```python
from build123d import *

# Parameters (mm, degrees)
SALIENTE_EXTRUIR1_DEPTH = 5
CROQUIS2_W              = 5
CROQUIS2_H              = 6.5
SALIENTE_EXTRUIR3_DEPTH = 5
REDONDEO1_R             = 3
REDONDEO2_R             = 2
REDONDEO3_R             = 1
CROQUIS4_R              = 1.75
CORTAR_EXTRUIR1_DEPTH   = 2.5
CROQUIS5_R              = 1
CORTAR_EXTRUIR2_DEPTH   = 2.5
CROQUIS6_R              = 0.75
CORTAR_EXTRUIR3_DEPTH   = 5


with BuildPart() as part:
    # Croquis1 → Saliente-Extruir1 (new body)
    with BuildSketch(Plane(origin=(0, 0, 0), x_dir=(0, 0, -1), z_dir=(1, 0, 0))):
        with BuildLine():
            Line((-13, 1.5), (13, 1.5))
            ThreePointArc((13, 1.5), (14.5, 0), (13, -1.5))
            Line((13, -1.5), (-13, -1.5))
            ThreePointArc((-13, -1.5), (-14.5, 0), (-13, 1.5))
        make_face()
    extrude(amount=SALIENTE_EXTRUIR1_DEPTH)

    # Croquis2 → Saliente-Extruir3 (add)
    with BuildSketch(Plane(origin=(5, 0, 0), x_dir=(0, 0, -1), z_dir=(1, 0, 0))):
        with Locations((-13, 0)):
            Rectangle(CROQUIS2_W, CROQUIS2_H)
        with Locations((13, 0)):
            Rectangle(CROQUIS2_W, CROQUIS2_H)
    extrude(amount=SALIENTE_EXTRUIR3_DEPTH)

    # Redondeo1
    redondeo1_edges = [part.edges().sort_by_distance(p)[0] for p in [
        (10, 3.25, 13),
        (10, 3.25, -13),
    ]]
    fillet(redondeo1_edges, radius=REDONDEO1_R)

    # Redondeo2
    redondeo2_edges = [part.edges().sort_by_distance(p)[0] for p in [
        (10, -3.25, 13),
        (10, -3.25, -13),
    ]]
    fillet(redondeo2_edges, radius=REDONDEO2_R)

    # Redondeo3
    redondeo3_edges = [part.edges().sort_by_distance(p)[0] for p in [
        (5, -3.25, 13),
        (5, -3.25, -13),
    ]]
    fillet(redondeo3_edges, radius=REDONDEO3_R)

    # Croquis4 → Cortar-Extruir1 (cut)
    with BuildSketch(Plane(origin=(0, 0, -15.5), x_dir=(-1, 0, 0), z_dir=(0, 0, -1))):
        with Locations((-7.5, 0)):
            Circle(CROQUIS4_R)
    cortar_extruir1 = extrude(amount=-CORTAR_EXTRUIR1_DEPTH, mode=Mode.SUBTRACT)

    # Croquis5 → Cortar-Extruir2 (cut)
    with BuildSketch(Plane(origin=(0, 0, -13), x_dir=(-1, 0, 0), z_dir=(0, 0, -1))):
        with Locations((-7.5, 0)):
            Circle(CROQUIS5_R)
    cortar_extruir2 = extrude(amount=-CORTAR_EXTRUIR2_DEPTH, mode=Mode.SUBTRACT)

    # Simetría2: Cortar-Extruir1, Cortar-Extruir2 across plane
    add(cortar_extruir1.mirror(Plane.XY), mode=Mode.SUBTRACT)
    add(cortar_extruir2.mirror(Plane.XY), mode=Mode.SUBTRACT)

    # Croquis6 → Cortar-Extruir3 (cut)
    with BuildSketch(Plane(origin=(0, 1.5, 0), x_dir=(1, 0, 0), z_dir=(0, 1, 0))):
        with Locations((1, 9)):
            Circle(CROQUIS6_R)
        with Locations((1, -9)):
            Circle(CROQUIS6_R)
    extrude(amount=-CORTAR_EXTRUIR3_DEPTH, mode=Mode.SUBTRACT)


solid = part.part
```
Input: part model. Units: mm. Frame: model coordinates. A direction names the side the tool comes from. Coordinates: 2 decimals unless noted, no trailing zeros. Order: outer loops, then holes, each group sorted by start corner. A loop starts at its lowest first (then second) coordinate and runs counter-clockwise, first axis right, second up. Notation, with made-up numbers: (7.5, 89.5) - (41.5, 89.5) arc R26 ccw to (41.5, 124.5) - close; hole circle Ø3 at (-5.75, -9). An arc over 180 degrees is marked (long way). Put each result on its own line as item: value.
1. Contact query for flat-ended pins moving along their axis: pin 1 Ø3 at (x, y) = (8, -1) entering from -Z; pin 2 Ø2 at (x, z) = (1, -9) entering from +Y; pin 3 Ø2.5 at (x, y) = (7.5, 0) entering from -Z; pin 4 Ø1 at (x, y) = (7, -0.5) entering from +Z. Output: stop coordinate, or through.
Report:
pin 1: stops at z = -15.5
pin 2: stops at y = 1.5
pin 3: stops at z = -13
pin 4: stops at z = 13
2. Cut plane A-A on x = 1. Return the cut outline in (y, z).
Report:
outline: (-1.5, -13) arc R1.5 ccw to (1.5, -13) - (1.5, -9.75) - (-1.5, -9.75) - close; (-1.5, -8.25) - (1.5, -8.25) - (1.5, 8.25) - (-1.5, 8.25) - close; (-1.5, 9.75) - (1.5, 9.75) - (1.5, 13) arc R1.5 ccw to (-1.5, 13) - close
3. Cut plane D-D on x = 7.5. Return the cut outline in (y, z).
Report:
outline: (-3.25, -15.5) - (-1.75, -15.5) - (-1.75, -13) - (-1, -13) - (-1, -10.5) - (-3.25, -10.5) - close; (-3.25, 10.5) - (-1, 10.5) - (-1, 13) - (-1.75, 13) - (-1.75, 15.5) - (-3.25, 15.5) - close; (1, -13) - (1.75, -13) - (1.75, -15.5) - (3.21, -15.5) - (3.21, -10.5) - (1, -10.5) - close; (1, 10.5) - (3.21, 10.5) - (3.21, 15.5) - (1.75, 15.5) - (1.75, 13) - (1, 13) - close
4. Reachability of faces 1 (the face through (2, -1.5, 0)), 2 (the face through (5, 0, 0)), 3 (the face through (2.5, 0, -14.5)) from +Z, -Z, +X, -X, +Y, -Y: full face, straight path, thin tool, end or side. Return the list, or none.
Report:
face 1: +Z, -Z, -X, -Y
face 2: +X, +Y, -Y
face 3: -Z, -X
5. Cut plane C-C on z = -9. Return the cut outline in (x, y).
Report:
outline: (0, -1.5) - (0.25, -1.5) - (0.25, 1.5) - (0, 1.5) - close; (1.75, -1.5) - (5, -1.5) - (5, 1.5) - (1.75, 1.5) - close
6. Cut plane B-B on y = 2.5. Return the cut outline in (x, z), then the cut area to 3 significant figures.
Report:
outline: (5, -15.5) - (8.98, -15.5) - (8.98, -10.5) - (5, -10.5) - close; (5, 10.5) - (8.98, 10.5) - (8.98, 15.5) - (5, 15.5) - close
area: 39.8 mm2
7. Draft query along X for faces 4 (the face through (6, 0, -13)), 5 (the face through (2, 1.5, 0)), 6 (the face through (9.1, 2.39, 12.96)). Return one class per face: pulls with the +X half, pulls with the -X half, needs draft (parallel to the pull), parting line crosses it, or undercut.
Report:
face 4: undercut
face 5: needs draft
face 6: pulls with the +X half
8. Line query: line 1 along Z through (x, y) = (6.25, 0.75); line 2 along Z through (x, y) = (8.5, 2.5); line 3 along Z through (x, y) = (1, 0.8). Output: solid intervals per line, ascending.
Report:
line 1: z = -13 to -10.5, 10.5 to 13
line 2: z = -15.5 to -10.5, 10.5 to 15.5
line 3: z = -14.27 to -9.75, -8.25 to 8.25, 9.75 to 14.27
